Input: part model. Units: mm. Frame: model coordinates. Give positions to 0.01 mm unless a question says otherwise; leave off trailing zeros. Order: outer loops, then holes, each group sorted by start corner. A loop starts at its lowest first (then second) coordinate and runs counter-clockwise, first axis right, second up. Notation, with made-up numbers: (-32, -30.5) -> (-28, -30.5) arc R18 ccw to (-28, -22.5) -> close; hole circle Ø8 at (47.25, 1.5). An arc over 180 degrees is marked (long way). Use a Markdown table: item, result. Add a question column.
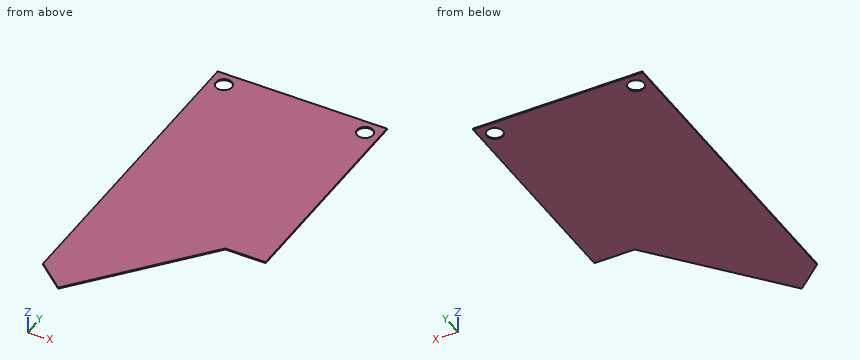
from build123d import *

# Parameters (mm, degrees)
SKETCH1_W           = 304.8
SKETCH1_H           = 635
BOSS_EXTRUDE1_DEPTH = 2.1082
SKETCH3_R           = 14.2875
CUT_EXTRUDE2_DEPTH  = 2.1082
SKETCH4_R           = 14.2875
CUT_EXTRUDE3_DEPTH  = 2.1082
CUT_EXTRUDE4_DEPTH  = 3.1082


with BuildPart() as part:
    # Sketch1 → Boss-Extrude1 (new body)
    with BuildSketch(Plane.XY):
        with Locations((101.6, -317.5)):
            Rectangle(SKETCH1_W, SKETCH1_H)
    extrude(amount=BOSS_EXTRUDE1_DEPTH)

    # Sketch3 → Cut-Extrude2 (cut)
    with BuildSketch(Plane(origin=(0, 0, 0), x_dir=(-1, 0, 0), z_dir=(0, 0, -1))):
        with Locations((25.4, -25.4)):
            Circle(SKETCH3_R)
    extrude(amount=-CUT_EXTRUDE2_DEPTH, mode=Mode.SUBTRACT)

    # Sketch4 → Cut-Extrude3 (cut)
    with BuildSketch(Plane(origin=(0, 0, 0), x_dir=(-1, 0, 0), z_dir=(0, 0, -1))):
        with Locations((-228.6, -25.4)):
            Circle(SKETCH4_R)
    extrude(amount=-CUT_EXTRUDE3_DEPTH, mode=Mode.SUBTRACT)

    # Sketch5 → Cut-Extrude4 (cut, through all)
    with BuildSketch(Plane(origin=(0, 0, 0), x_dir=(-1, 0, 0), z_dir=(0, 0, -1))):
        Polygon((-254, -635), (-254, -393.7), (-181.170170025, -393.7), (0, -609.6), (50.8, -566.973738736), (50.8, -635), align=None)
    extrude(amount=-CUT_EXTRUDE4_DEPTH, mode=Mode.SUBTRACT)


solid = part.part
Q1. Section query D-D (x = -25.4). Return loops of the section in (y, z), plus the area to 3 significant figures.
Q2. Section query C-C (z = 0.65). Return loops of the section in (x, y) (1 decimal), plus the area to 3 significant figures.
Q3. First-contact query: pin 1 (1 mm diameter, centred on x = 157.5, z = 1, fed in from -Y); pin 2 (23 mm diameter, centred on x = 228.6, y = -25.4, fed in from -Z); pin 3 (0.6 mm diameter, centred on x = 213.5, z = 1.5, fed in from -Y). Flat tips, straight axial feed; report the tip coordinate or a pass-through.
Q4. Section query B-B (y = -25.4). Return loops of the section in (x, z).
Q5. Section query A-A (x = 228.6). Return loops of the section in (y, z), plus the area to 3 significant figures.
Q6. Ray query, line 1 (Y direction, x = 228.6, z = 1.2); line 2 (Y direction, x = 207.5, z = 0.7); line 3 (Y direction, x = -25.4, z = 1.2). Return the intervals inside material, ascending.
Solution:
| question | item | result |
|---|---|---|
| 1 | outline | (-588.29, 0) -> (-39.69, 0) -> (-39.69, 2.11) -> (-588.29, 2.11) -> close; (-11.11, 0) -> (0, 0) -> (0, 2.11) -> (-11.11, 2.11) -> close |
| 1 | area | 1,180 mm² |
| 2 | outline | (-50.8, -567) -> (0, -609.6) -> (181.2, -393.7) -> (254, -393.7) -> (254, 0) -> (-50.8, 0) -> close; hole circle Ø28.6 at (-25.4, -25.4); hole circle Ø28.6 at (228.6, -25.4) |
| 2 | area | 148,000 mm² |
| 3 | pin 1 | stops at y = -422.5 |
| 3 | pin 2 | passes through |
| 3 | pin 3 | stops at y = -393.7 |
| 4 | outline | (-50.8, 0) -> (-39.69, 0) -> (-39.69, 2.11) -> (-50.8, 2.11) -> close; (-11.11, 0) -> (214.31, 0) -> (214.31, 2.11) -> (-11.11, 2.11) -> close; (242.89, 0) -> (254, 0) -> (254, 2.11) -> (242.89, 2.11) -> close |
| 5 | outline | (-393.7, 0) -> (-39.69, 0) -> (-39.69, 2.11) -> (-393.7, 2.11) -> close; (-11.11, 0) -> (0, 0) -> (0, 2.11) -> (-11.11, 2.11) -> close |
| 5 | area | 770 mm² |
| 6 | line 1 | y = -393.7 to -39.69, -11.11 to 0 |
| 6 | line 2 | y = -393.7 to 0 |
| 6 | line 3 | y = -588.29 to -39.69, -11.11 to 0 |
